from build123d import *

# Parameters (mm, degrees)
F0_R        = 10.6794819522
F1_DEPTH    = 6.35
F2_R        = 10.6995432546
F3_DEPTH    = 1.5875
F4_T1_DEPTH = 6.35
F5_T1_DEPTH = 6.35


# Not quite as in the source:
# - a fillet or chamfer that OpenCascade refuses, or shapes differently, is made with other operations: its cross-section is extruded or revolved along the edge and cut away or added


with BuildPart() as f1:
    # F0 (on Top) → F1 (new body)
    with BuildSketch(Plane.XY):
        with BuildLine():
            Line((50.8, 3.175), (12.2967221242, 3.175))
            ThreePointArc((12.2967221242, 3.175), (-12.7, 0), (12.2967221242, -3.175))
            Line((12.2967221242, -3.175), (50.8, -3.175))
            Line((50.8, -3.175), (50.8, 3.175))
        make_face()
        Circle(F0_R, mode=Mode.SUBTRACT)
    extrude(amount=F1_DEPTH)

    # F2 (on face) → F3 (join)
    with BuildSketch(Plane.XY.offset(6.35)):
        with BuildLine():
            ThreePointArc((12.2967221242, -3.175), (12.5987771426, -1.6002545145), (12.7, 0))
            ThreePointArc((12.7, 0), (12.5987771426, 1.6002545145), (12.2967221242, 3.175))
            ThreePointArc((12.2967221242, 3.175), (-12.7, 0), (12.2967221242, -3.175))
        make_face()
        Circle(F2_R, mode=Mode.SUBTRACT)
    extrude(amount=F3_DEPTH)

    # F4: fillet of radius 5.08 on 1 edges, made by hand

    # F4_s2 → F4_t1 (join)
    with BuildSketch(Plane.XY):
        with BuildLine():
            ThreePointArc((15.7474878949, -3.175), (13.1183381138, -3.908280383), (11.2482056392, -5.8964285714))
            ThreePointArc((11.2482056392, -5.8964285714), (11.8508417091, -4.5659118242), (12.2967221242, -3.175))
            Line((12.2967221242, -3.175), (15.7474878949, -3.175))
        make_face()
    extrude(amount=F4_T1_DEPTH)

    # F5: fillet of radius 5.08 on 1 edges, made by hand

    # F5_s2 → F5_t1 (join)
    with BuildSketch(Plane.XY):
        with BuildLine():
            ThreePointArc((15.7474878949, 3.175), (13.1183381138, 3.908280383), (11.2482056392, 5.8964285714))
            ThreePointArc((11.2482056392, 5.8964285714), (11.8508417091, 4.5659118242), (12.2967221242, 3.175))
            Line((12.2967221242, 3.175), (15.7474878949, 3.175))
        make_face()
    extrude(amount=F5_T1_DEPTH)


solid = f1.part
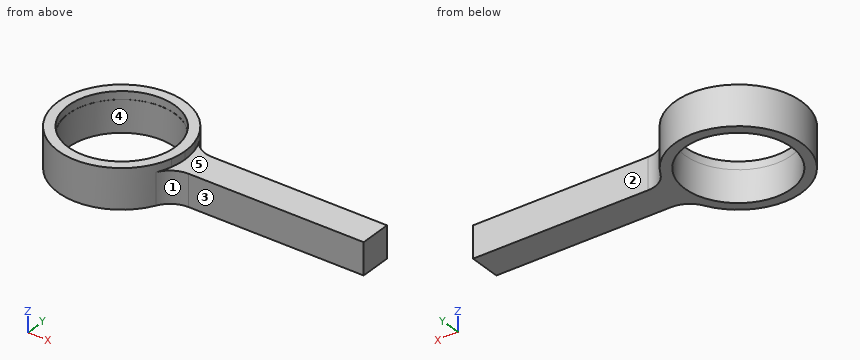
Read the model definition and answer for the solid it produces. Units are mm, in the model's axes. Face numbers are marked on the shaded views. A direction names the side the tool comes from. Give positions to 0.01 mm unless a question says otherwise; leave off trailing zeros. Loops run counter-clockwise (first coordinate to the right, second up) from the corner with the lowest first, then second, coordinate; pieces in that order, holes last. Notation, with made-up numbers: (-35.75, 43) - (-25.75, 43) arc R24 cw to (-25.75, 68) - close; hole circle Ø10 at (81.5, 49). An arc over 180 degrees is marked (long way). Answer as CSV lines item,"result". Start each with the question number.
1) Find section B-B (z = 4.5). Write down the section's boundary in (x, y) (3 decimals).
2) Determine the mould class of the marked faces 3, 4 and 5 for opening direction Y: released by +Y, released by -Y, zero draft, split by the parting line, or undercut.
3) Which of the six approach directions +Z, -Z, +X, -X, +Y, -Y give full straight-line access (tool end or side, diameter ignored) to the marked faces 1 and 2?
4) Each of these flat-tipped pins is pushed along its axis until it touches: pin 1 Ø5 at (x, y) = (-5, 8.5) entering from +Z; pin 2 Ø13 at (x, y) = (35.5, 1.5) entering from +Z; pin 3 Ø1.5 at (x, z) = (15, 1.5) entering from +Y. Where does it stop, or does it pass through?
5) Straight lines are drawn through the part: L1, parallel to Y at x = 0, z = 1.75; L2, parallel to Z at x = 22, y = -1.5; L3, parallel to Y at x = 39.5, z = 1 (3 decimals). For each, find the intervals that lie inside material, in ascending order. Write a range as from..to.
6) Find section D-D (x = 9.5). Write down the section's boundary in (y, z).
Findings below:
1,outline,"(11.248, -5.896) arc R5.08 cw to (15.747, -3.175) - (50.8, -3.175) - (50.8, 3.175) - (15.747, 3.175) arc R5.08 cw to (11.248, 5.896) arc R12.7 ccw (long way) to start; hole circle Ø21.359 at (0, 0)"
2,face 3,"released by -Y"
2,face 4,"undercut"
2,face 5,"zero draft"
3,face 1,"+Z, -Z, +X, -Y"
3,face 2,"+Z, -Z, +X, +Y"
4,pin 1,"z = 7.94"
4,pin 2,"z = 6.35"
4,pin 3,"y = 3.4"
5,L1,"-12.7..-10.68, 10.68..12.7"
5,L2,"0..6.35"
5,L3,"-3.175..3.175"
6,outline,"(-8.43, 0) - (-4.88, 0) - (-4.88, 6.35) - (-4.92, 6.35) - (-4.92, 7.94) - (-8.43, 7.94) - close; (4.88, 0) - (8.43, 0) - (8.43, 7.94) - (4.92, 7.94) - (4.92, 6.35) - (4.88, 6.35) - close"
